Autodesk Inventor part; units mm, degrees
ref_plane "YZ Plane" through (0, 0, 0) normal (1, 0, 0) x (0, 1, 0)
ref_plane "XZ Plane" through (0, 0, 0) normal (0, 1, 0) x (-1, 0, 0)
ref_plane "XY Plane" through (0, 0, 0) normal (0, 0, 1) x (1, 0, 0)
sketch "Esboço1" plane through (0, 0, 0) normal (0, 0, 1) x (1, 0, 0)
  circle A0 centre (0, 0) radius 25
  circle A1 centre (0, 0) radius 30
  dimension "d0" = 50
  dimension "d1" = 60
extrude "Extrusão1" add sketch "Esboço1" along normal blind 20
extrude "Extrusão2" add sketch "Esboço1" along normal blind 5 contours A0
sketch "Esboço2" plane through (0, 0, 0) normal (0, 0, -1) x (-1, 0, 0)
  circle A0 centre (0, 0) radius 15
  dimension "d6" = 30
extrude "Extrusão3" add sketch "Esboço2" along normal blind 15
properties part number "Engrenagem"
Part model, mm, in its own coordinate system. A direction names the side the tool comes from. Round coordinates to 2 decimals unless told otherwise and drop trailing zeros. Write each loop counter-clockwise with the first axis right and the second up, starting at its lowest first coordinate (ties: lowest second). Pieces come first, ordered by that corner, then holes. Notation, with made-up numbers: M 21.25,-33.5 L 33.25,-33.5 A27 cw 33.25,-7.5 Z; hole C 59,63 d4. An arc over 180 degrees is marked long. Return JSON: item names as keys, results as strings. Group by question number.
(1) Saw through at D-D on x = -24. Write the cut outline in (y, z).
(2) Two-plate mould, pull along Y, no slides. Class faces 4 (the face through (14.985, -0.66, -7.395)), 5 (the face through (23.846, -7.509, 12.395)), 6 (the face through (0, 0, -15)): +Y half, -Y half, draft (parallel to the pull), parting line (faces both ways), or undercut.
(3) Pin check, flat tips, straight feed: pin 1 Ø3 at (y, z) = (-12.5, 15) entering from +X; pin 2 Ø8 at (y, z) = (-10.5, 2.5) entering from +X; pin 3 Ø3 at (y, z) = (11.5, -11.5) entering from +X. Stop position of each tip, or through.
(4) Drill centre lines: probe 1 along Y at (x, z) = (0, 11); probe 2 along Z at (x, y) = (-4, 3); probe 3 along Y at (x, z) = (-17.5, 17). Where is each one in solid material? Low to high.
(5) Saw through at C-C on z = 2.5. Write the cut outline in (x, y).
(6) Which spindle directions (+Z, -Z, +X, -X, +Y, -Y) get a long thin tool onto all of the face, cutting with end or side? Do faces 1 (the face through (-29.97, -1.32, 9.86)), 2 (the face through (6, 14, 0)), 3 (the face through (0, 0, 5)). Say none if no direction does.
(7) Saw through at A-A on x = 0. Write the cut outline in (y, z), then the cut area to 3 significant figures.
Returned:
{
 "1": {"outline": "M -18,0 L 18,0 L 18,20 L 7,20 L 7,5 L -7,5 L -7,20 L -18,20 Z"},
 "2": {"face 4": "parting line", "face 5": "undercut", "face 6": "draft"},
 "3": {"pin 1": "x = 27.91", "pin 2": "x = 29.29", "pin 3": "x = 11.18"},
 "4": {"probe 1": "-30 to -25, 25 to 30", "probe 2": "-15 to 5", "probe 3": "-24.37 to -17.85, 17.85 to 24.37"},
 "5": {"outline": "C 0,0 d60"},
 "6": {"face 1": "+Z, -Z", "face 2": "-Z", "face 3": "+Z"},
 "7": {"outline": "M -30,0 L -15,0 L -15,-15 L 15,-15 L 15,0 L 30,0 L 30,20 L 25,20 L 25,5 L -25,5 L -25,20 L -30,20 Z", "area": "900 mm²"}
}
